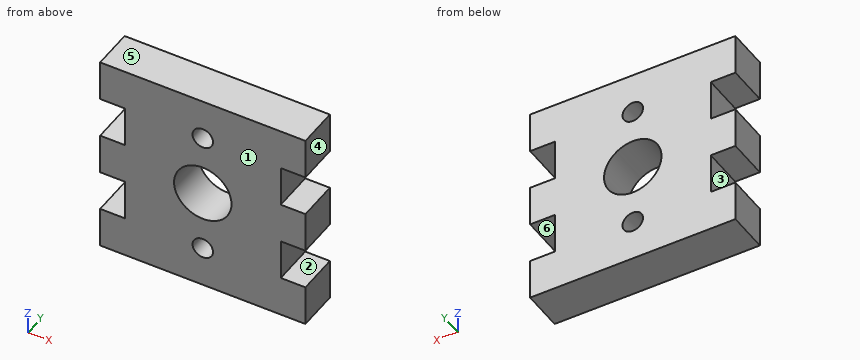
from build123d import *

# Parameters (mm, degrees)
SKETCH1_W           = 25
SKETCH1_H           = 25
SKETCH1_R           = 3.5
BOSS_EXTRUDE1_DEPTH = 5
SKETCH2_W           = 3
SKETCH2_H           = 5
CUT_EXTRUDE1_DEPTH  = 15
SKETCH3_R           = 1.25
SKETCH3_R_2         = 3.402319191
CUT_EXTRUDE2_DEPTH  = 5


with BuildPart() as part:
    # Sketch1 → Boss-Extrude1 (new body)
    with BuildSketch(Plane(origin=(0, 0, 0), x_dir=(1, 0, 0), z_dir=(0, 1, 0))):
        with Locations((1.342975207, -1.859504132)):
            Rectangle(SKETCH1_W, SKETCH1_H)
        with Locations(Location((1.342975207, -1.859504132, 0), (0, 0, 270))):
            Circle(SKETCH1_R, mode=Mode.SUBTRACT)
    extrude(amount=BOSS_EXTRUDE1_DEPTH)

    # Sketch2 → Cut-Extrude1 (cut)
    with BuildSketch(Plane(origin=(0, 5, 0), x_dir=(1, 0, 0), z_dir=(0, 1, 0))):
        with Locations((-9.657024793, 3.140495868)):
            Rectangle(SKETCH2_W, SKETCH2_H)
        with Locations((-9.657024793, -6.859504132)):
            Rectangle(SKETCH2_W, SKETCH2_H)
        with Locations((12.342975207, -6.859504132)):
            Rectangle(SKETCH2_W, SKETCH2_H)
        with Locations((12.342975207, 3.140495868)):
            Rectangle(SKETCH2_W, SKETCH2_H)
    extrude(amount=-CUT_EXTRUDE1_DEPTH, mode=Mode.SUBTRACT)

    # Sketch3 → Cut-Extrude2 (cut)
    with BuildSketch(Plane(origin=(0, 5, 0), x_dir=(1, 0, 0), z_dir=(0, 1, 0))):
        with Locations(Location((1.342975207, 5.640495868, 0), (0, 0, 270))):
            Circle(SKETCH3_R)
        with Locations(Location((1.342975207, -9.359504132, 0), (0, 0, 270))):
            Circle(SKETCH3_R)
        with Locations((1.342975207, -1.859504132)):
            Circle(SKETCH3_R_2)
    extrude(amount=-CUT_EXTRUDE2_DEPTH, mode=Mode.SUBTRACT)


solid = part.part
CAD build for the part. Positions are in the model's coordinates, mm. Face numbers are marked on the shaded views. A direction names the side the tool comes from. Round coordinates to 2 decimals unless told otherwise and drop trailing zeros. Order: outer loops, then holes, each group sorted by start corner. A loop starts at its lowest first (then second) coordinate and runs counter-clockwise, first axis right, second up. Notation, with made-up numbers: M 36,-22.75 L 76,-22.75 A16 cw 76,5.25 Z; hole C 15,-13.75 d4. An arc over 180 degrees is marked long. Use one line per item in the form item = value.
Q1. Saw through at D-D on z = -3.5. Give the cut face in (x, y).
Recorded:
outline = M -8.16,0 L 10.84,0 L 10.84,5 L -8.16,5 Z
Q2. Saw through at C-C on x = -0.5. Give the cut face in (y, z), then the cut area to 3 significant figures.
Recorded:
outline = M 0,-10.64 L 5,-10.64 L 5,-1.12 L 0,-1.12 Z; M 0,4.83 L 5,4.83 L 5,14.36 L 0,14.36 Z
area = 95.2 mm^2
Q3. Flat gauge pins, fed straight in: P1, Ø3, axis at x = 5, z = -2.5, coming from the -Y side; P2, Ø1.5, axis at y = 3, z = -2.5, coming from the +X side; P3, Ø1.5, axis at x = 1.34, z = 9.36, coming from the -Y side. Where does each tip first touch, or does it go through?
Recorded:
P1 = 0
P2 = 10.84
P3 = through
Q4. Two-plate mould, pull along Z, no slides. Class the marked faces 4, 5 and 6: +Z half, -Z half, draft (parallel to the pull), parting line (faces both ways), or undercut.
Recorded:
face_4 = draft
face_5 = +Z half
face_6 = undercut
Q5. Saw through at A-A on z = 0. Give the cut face in (x, y).
Recorded:
outline = M -11.16,0 L -1.62,0 L -1.62,5 L -11.16,5 Z; M 4.31,0 L 13.84,0 L 13.84,5 L 4.31,5 Z
Q6. Which spindle directions (+Z, -Z, +X, -X, +Y, -Y) get a long thin tool onto all of the face, cutting with end or side? Do the marked faces 1, 2 and 3. Say none if no direction does.
Recorded:
face_1 = +Z, -Z, +X, -X, -Y
face_2 = +X, +Y, -Y
face_3 = -X, +Y, -Y
Q7. Probe L1, parallel to Z at x = 11.75, y = 1.3; L2, parallel to X at y = 0.85, z = 2; L3, parallel to Z at x = 0.25, y = 1.85. List the from-to ranges inside material, lowest first.
Recorded:
L1 = -10.64 to -5.64, -0.64 to 4.36, 9.36 to 14.36
L2 = -11.16 to -2.15, 4.84 to 13.84
L3 = -10.64 to -6.25, -5.03 to -1.47, 5.18 to 8.75, 9.97 to 14.36
Q8. Saw through at B-B on y = 3.75. Give the cut face in (x, z), then the cut area to 3 significant figures.
Recorded:
outline = M -11.16,-10.64 L 13.84,-10.64 L 13.84,-5.64 L 10.84,-5.64 L 10.84,-0.64 L 13.84,-0.64 L 13.84,4.36 L 10.84,4.36 L 10.84,9.36 L 13.84,9.36 L 13.84,14.36 L -11.16,14.36 L -11.16,9.36 L -8.16,9.36 L -8.16,4.36 L -11.16,4.36 L -11.16,-0.64 L -8.16,-0.64 L -8.16,-5.64 L -11.16,-5.64 Z; hole C 1.34,1.86 d7; hole C 1.34,-5.64 d2.5; hole C 1.34,9.36 d2.5
area = 517 mm^2
